Part model, mm, in its own coordinate system. A direction names the side the tool comes from. Round coordinates to 2 decimals unless told otherwise and drop trailing zeros. Write each loop counter-clockwise with the first axis right and the second up, starting at its lowest first coordinate (ties: lowest second). Pieces come first, ordered by that corner, then holes. Notation, with made-up numbers: (47, -21.5) -> (100, -21.5) arc R22 cw to (100, -5.5) -> close; hole circle Ø2 at (78.25, 47.25). An arc over 180 degrees is marked (long way). Return JSON: item names as keys, results as strings. Group by question number.
(1) Saw through at D-D (y = 7.75). List the corners of the cut face in (x, z).
(2) Saw through at B-B (x = 7.5). List the corners of the cut face in (y, z), plus the area to 3 significant figures.
(3) Mould opens along Y. For faces 1 (the flat face through (25, 10, 1)), 2 (the flat face through (-25, 10, 1)), 3 (the flat face through (-26.6, 3, 1)) say: +Y half, -Y half, draft (parallel to the pull), parting line (faces both ways), or undercut.
(4) Saw through at A-A (x = -3.75). List the corners of the cut face in (y, z).
(5) Tool access for faces 4 (the flat face through (-23.6, 8, 1)), 5 (the flat face through (23.6, 12, 1)), 6 (the flat face through (23.6, 2, 1)), 7 (the flat face through (26.6, -13, 1)), 8 (the cylindrical face through (-1.5, 0.07, 1.52)): list every direction of +Z, -Z, +X, -X, +Y, -Y with a clear straight run to the whole face (end or side of a thin tool).
(6) Drill centre lines: L1, parallel to Y at x = 3.75, z = 1.45; L2, parallel to Y at x = 0, z = 2.1; L3, parallel to Y at x = 4, z = 0.5. Where is each one in solid material? Low to high. Write a range as from..to.
(7) Saw through at C-C (z = 1.3). State how many separate pieces and enclosed holes the cut face has, plus the area to 3 significant figures.
(8) Drop flat-ended pins along their axis: pin 1 Ø0.9 at (x, z) = (-25.5, 1.5) entering from -Y; pin 2 Ø1.5 at (x, z) = (24.5, 1.5) entering from +Y; pin 3 Ø1.5 at (y, z) = (8, 2) entering from -X. Give the stop position or say it passes through.
from build123d import *

# Parameters (mm, degrees)
SALIENTE_EXTRUIR1_DEPTH = 3
CORTAR_EXTRUIR1_REACH   = 32.685
CROQUIS2_R              = 1.5
CROQUIS2_R_2            = 0.75


with BuildPart() as part:
    # Croquis1 → Saliente-Extruir1 (new body)
    with BuildSketch(Plane.XY):
        Polygon((26.6, 5), (26.6, 10), (23.6, 10), (23.6, 15), (-26.6, 15), (-26.6, 10), (-23.6, 10), (-23.6, 5), (-26.6, 5), (-26.6, 0), (-23.6, 0), (-23.6, -5), (-26.6, -5), (-26.6, -10), (-23.6, -10), (-23.6, -15), (26.6, -15), (26.6, -10), (23.6, -10), (23.6, -5), (26.6, -5), (26.6, 0), (23.6, 0), (23.6, 5), align=None)
    extrude(amount=SALIENTE_EXTRUIR1_DEPTH)

    # Croquis2 → Cortar-Extruir1 (cut, up to next)
    with BuildSketch(Plane.XY.offset(3), mode=Mode.PRIVATE) as cortar_extruir1_sk1:
        Circle(CROQUIS2_R)
    cortar_extruir1_tool1 = extrude(cortar_extruir1_sk1.sketch, amount=-CORTAR_EXTRUIR1_REACH, mode=Mode.PRIVATE) & part.part
    # Croquis2 → Cortar-Extruir1 (cut, up to next)
    with BuildSketch(Plane.XY.offset(3), mode=Mode.PRIVATE) as cortar_extruir1_sk2:
        with Locations((7.5, 0)):
            Circle(CROQUIS2_R_2)
    cortar_extruir1_tool2 = extrude(cortar_extruir1_sk2.sketch, amount=-CORTAR_EXTRUIR1_REACH, mode=Mode.PRIVATE) & part.part
    # Croquis2 → Cortar-Extruir1 (cut, up to next)
    with BuildSketch(Plane.XY.offset(3), mode=Mode.PRIVATE) as cortar_extruir1_sk3:
        with Locations((3.75, -6.495190528)):
            Circle(CROQUIS2_R_2)
    cortar_extruir1_tool3 = extrude(cortar_extruir1_sk3.sketch, amount=-CORTAR_EXTRUIR1_REACH, mode=Mode.PRIVATE) & part.part
    # Croquis2 → Cortar-Extruir1 (cut, up to next)
    with BuildSketch(Plane.XY.offset(3), mode=Mode.PRIVATE) as cortar_extruir1_sk4:
        with Locations((-3.75, -6.495190528)):
            Circle(CROQUIS2_R_2)
    cortar_extruir1_tool4 = extrude(cortar_extruir1_sk4.sketch, amount=-CORTAR_EXTRUIR1_REACH, mode=Mode.PRIVATE) & part.part
    # Croquis2 → Cortar-Extruir1 (cut, up to next)
    with BuildSketch(Plane.XY.offset(3), mode=Mode.PRIVATE) as cortar_extruir1_sk5:
        with Locations((-7.5, 0)):
            Circle(CROQUIS2_R_2)
    cortar_extruir1_tool5 = extrude(cortar_extruir1_sk5.sketch, amount=-CORTAR_EXTRUIR1_REACH, mode=Mode.PRIVATE) & part.part
    # Croquis2 → Cortar-Extruir1 (cut, up to next)
    with BuildSketch(Plane.XY.offset(3), mode=Mode.PRIVATE) as cortar_extruir1_sk6:
        with Locations((-3.75, 6.495190528)):
            Circle(CROQUIS2_R_2)
    cortar_extruir1_tool6 = extrude(cortar_extruir1_sk6.sketch, amount=-CORTAR_EXTRUIR1_REACH, mode=Mode.PRIVATE) & part.part
    # Croquis2 → Cortar-Extruir1 (cut, up to next)
    with BuildSketch(Plane.XY.offset(3), mode=Mode.PRIVATE) as cortar_extruir1_sk7:
        with Locations((3.75, 6.495190528)):
            Circle(CROQUIS2_R_2)
    cortar_extruir1_tool7 = extrude(cortar_extruir1_sk7.sketch, amount=-CORTAR_EXTRUIR1_REACH, mode=Mode.PRIVATE) & part.part
    add(cortar_extruir1_tool1.solids().sort_by_distance((0, 0, 3))[0], mode=Mode.SUBTRACT)
    add(cortar_extruir1_tool2.solids().sort_by_distance((7.5, 0, 3))[0], mode=Mode.SUBTRACT)
    add(cortar_extruir1_tool3.solids().sort_by_distance((3.75, -6.495191, 3))[0], mode=Mode.SUBTRACT)
    add(cortar_extruir1_tool4.solids().sort_by_distance((-3.75, -6.495191, 3))[0], mode=Mode.SUBTRACT)
    add(cortar_extruir1_tool5.solids().sort_by_distance((-7.5, 0, 3))[0], mode=Mode.SUBTRACT)
    add(cortar_extruir1_tool6.solids().sort_by_distance((-3.75, 6.495191, 3))[0], mode=Mode.SUBTRACT)
    add(cortar_extruir1_tool7.solids().sort_by_distance((3.75, 6.495191, 3))[0], mode=Mode.SUBTRACT)


solid = part.part
Computed values:
{
 "1": {"outline": "(-23.6, 0) -> (26.6, 0) -> (26.6, 3) -> (-23.6, 3) -> close"},
 "2": {"outline": "(-15, 0) -> (-0.75, 0) -> (-0.75, 3) -> (-15, 3) -> close; (0.75, 0) -> (15, 0) -> (15, 3) -> (0.75, 3) -> close", "area": "85.5 mm2"},
 "3": {"face 1": "+Y half", "face 2": "undercut", "face 3": "draft"},
 "4": {"outline": "(-15, 0) -> (-7.25, 0) -> (-7.25, 3) -> (-15, 3) -> close; (-5.75, 0) -> (5.75, 0) -> (5.75, 3) -> (-5.75, 3) -> close; (7.25, 0) -> (15, 0) -> (15, 3) -> (7.25, 3) -> close"},
 "5": {"face 4": "+Z, -Z, -X", "face 5": "+Z, -Z, +X, +Y", "face 6": "+Z, -Z, +X", "face 7": "+Z, -Z, +X, +Y, -Y", "face 8": "+Z, -Z"},
 "6": {"L1": "-15..-7.25, -5.75..5.75, 7.25..15", "L2": "-15..-1.5, 1.5..15", "L3": "-15..-7.2, -5.79..5.79, 7.2..15"},
 "7": {"separate pieces": "1", "enclosed holes": "7", "area": "1,490 mm2"},
 "8": {"pin 1": "y = -10", "pin 2": "y = 10", "pin 3": "x = -23.6"}
}
